Verification items for the finished model (mm, model axes). Face numbers are marked on the shaded views. Give positions to 0.01 mm unless a question says otherwise; leave off trailing zeros. Write each loop counter-clockwise with the first axis right and the second up, starting at its lowest first coordinate (ties: lowest second). Pieces come first, ordered by that corner, then holes.
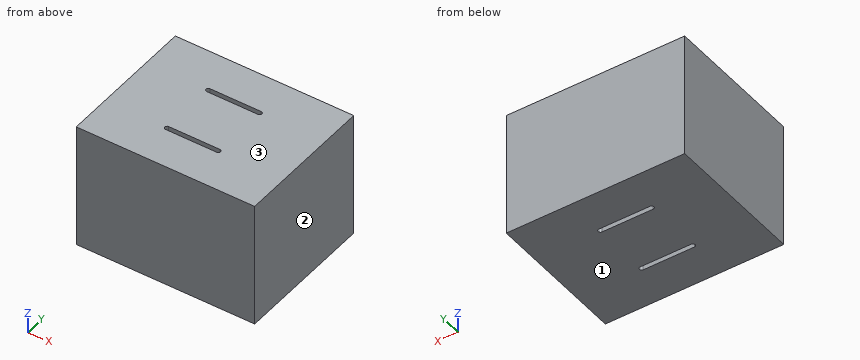
from build123d import *

# Parameters (mm, degrees)
SKETCH1_W           = 53.8
SKETCH1_H           = 37.83
BOSS_EXTRUDE1_DEPTH = 42.85
CUT_EXTRUDE1_DEPTH  = 2


with BuildPart() as part:
    # Sketch1 → Boss-Extrude1 (new body)
    with BuildSketch(Plane(origin=(0, 0, 0), x_dir=(1, 0, 0), z_dir=(0, 1, 0))):
        Rectangle(SKETCH1_W, SKETCH1_H)
    extrude(amount=BOSS_EXTRUDE1_DEPTH)

    # Sketch2 → Cut-Extrude1 (cut)
    with BuildSketch(Plane(origin=(0, 0, -18.915), x_dir=(-1, 0, 0), z_dir=(0, 0, -1))):
        with BuildLine():
            Line((-7.225, 31.025), (8.225, 31.025))
            ThreePointArc((8.225, 31.025), (8.9, 30.35), (8.225, 29.675))
            Line((8.225, 29.675), (-7.225, 29.675))
            ThreePointArc((-7.225, 29.675), (-7.9, 30.35), (-7.225, 31.025))
        make_face()
        with BuildLine():
            Line((-7.225, 13.175), (8.225, 13.175))
            ThreePointArc((8.225, 13.175), (8.9, 12.5), (8.225, 11.825))
            Line((8.225, 11.825), (-7.225, 11.825))
            ThreePointArc((-7.225, 11.825), (-7.9, 12.5), (-7.225, 13.175))
        make_face()
    cut_extrude1 = extrude(amount=-CUT_EXTRUDE1_DEPTH, mode=Mode.SUBTRACT)

    # Mirror1: Cut-Extrude1 across plane
    add(cut_extrude1.mirror(Plane(origin=(0, 0, 0), x_dir=(1, 0, 0), z_dir=(0, 0, -1))), mode=Mode.SUBTRACT)


solid = part.part
Item 1: Release check for a two-part mould opening along Z. For the marked faces 1, 2 and 3 record: released by +Z, released by -Z, zero draft, split by the parting line, or undercut.
Answer key:
face 1: released by -Z
face 2: zero draft
face 3: released by +Z
Item 2: Sectioned sample at A-A on y = 12.5. Record the cut outline in (x, z) (3 decimals), then the cut area to 3 significant figures.
Answer key:
outline: (-26.9, -18.915) - (-8.9, -18.915) - (-8.9, -16.915) - (7.9, -16.915) - (7.9, -18.915) - (26.9, -18.915) - (26.9, 18.915) - (7.9, 18.915) - (7.9, 16.915) - (-8.9, 16.915) - (-8.9, 18.915) - (-26.9, 18.915) - close
area: 1,970 mm2
Item 3: Depth check by flat-ended pin: pin 1 (1.1 mm diameter, centred on x = -2.5, y = 12.5, fed in from +Z) (3 decimals); pin 2 (0.7 mm diameter, centred on x = -4.5, y = 30.5, fed in from -Z) (3 decimals). Enter the tip coordinate at first touch or a pass-through.
Answer key:
pin 1: stops at z = 16.915
pin 2: stops at z = -16.915
Item 4: Scan line: line 1 along Z through (x, y) = (-6, 12.5) (3 decimals). Record every from-to range of solid material in increasing order.
Answer key:
line 1: z = -16.915 to 16.915
